Model file for the job. Use its own axes, mm. A direction names the side the tool comes from. Round coordinates to 2 decimals unless told otherwise and drop trailing zeros. Order: outer loops, then holes, each group sorted by start corner. A loop starts at its lowest first (then second) coordinate and runs counter-clockwise, first axis right, second up. Notation, with made-up numbers: (-34.75, 69) - (5.25, 69) arc R4 ccw to (5.25, 75) - close; hole circle Ø2 at (68.5, 19). An arc over 180 degrees is marked (long way). Put each result on its own line as item: value. Start each with the question number.
Item 1: Saw through at B-B on z = -3.5. List the corners of the cut face in (x, y).
Item 2: Mould opens along X. For faces 1 (the face through (-13.268, 9.392, -33.573)), 2 (the face through (32.187, 9.392, -20.386)), 3 (the face through (-36.225, 9.392, -11.806)), 4 (the face through (-11.837, 9.658, -16.703)) say: pulls with the +X half, pulls with the -X half, needs draft (parallel to the pull), parting line crosses it, or undercut.
Item 3: Which spindle directions (+Z, -Z, +X, -X, +Y, -Y) get a long thin tool onto all of the face, cutting with end or side? Do faces 5 (the face through (4.741, 9.392, 37.804)), 6 (the face through (37.1, 9.39, 0.34)), 7 (the face through (32.35, 9.39, 18.17)), 8 (the face through (36.246, 9.392, -11.741)), 9 (the face through (20, 10, -1.9)). Say none if no direction does.
Item 4: Probe probe 1 along Z at (x, y) = (-18, 15.25); probe 2 along Z at (x, y) = (1, 11.5); probe 3 along X at (y, z) = (18, 31.5). List the from-to ranges inside material, lowest first.
Item 5: Pin check, flat tips, straight feed: pin 1 Ø3 at (y, z) = (11.5, -21) entering from -X; pin 2 Ø4 at (x, y) = (21, 13) entering from +Z; pin 3 Ø10 at (y, z) = (15, 20) entering from -X; pin 4 Ø5 at (x, y) = (1, 7.5) entering from +Z. Stop position of each tip, or through.
Item 6: Saw through at A-A on x = 4. List the corners of the cut face in (y, z), plus the area to 3 significant figures.
```python
from build123d import *

# Parameters (mm, degrees)
SKETCH1_R           = 38.1
BOSS_EXTRUDE1_DEPTH = 19.05
CUT_EXTRUDE1_DEPTH  = 33
CIRPATTERN1_COUNT   = 25
SKETCH3_R           = 18
CUT_EXTRUDE2_DEPTH  = 28
CUT_EXTRUDE8_DEPTH  = 23
CIRPATTERN2_COUNT   = 12


with BuildPart() as part:
    # Sketch1 → Boss-Extrude1 (new body)
    with BuildSketch(Plane(origin=(0, 0, 0), x_dir=(1, 0, 0), z_dir=(0, 1, 0))):
        with Locations(Location((0, 0, 0), (0, 0, 90))):
            Circle(SKETCH1_R)
    extrude(amount=BOSS_EXTRUDE1_DEPTH)

    # Sketch2 → Cut-Extrude1 (cut)
    with BuildSketch(Plane.XZ):
        Polygon((0, 38.1), (-2.36, 38.1), (-1.66, 36.1), (0, 36.1), (1.66, 36.1), (2.36, 38.1), align=None)
    cut_extrude1 = extrude(amount=-CUT_EXTRUDE1_DEPTH, mode=Mode.SUBTRACT)

    # CirPattern1: Cut-Extrude1 ×25 about axis
    cirpattern1_axis = Axis((0, 0, 0), (0, 1, 0))
    for i in range(1, CIRPATTERN1_COUNT):
        add(cut_extrude1.rotate(cirpattern1_axis, i * 360 / CIRPATTERN1_COUNT), mode=Mode.SUBTRACT)

    # Sketch3 → Cut-Extrude2 (cut)
    with BuildSketch(Plane(origin=(0, 19.05, 0), x_dir=(1, 0, 0), z_dir=(0, 1, 0))):
        with Locations(Location((0, 0, 0), (0, 0, 270))):
            Circle(SKETCH3_R)
    extrude(amount=-CUT_EXTRUDE2_DEPTH, mode=Mode.SUBTRACT)

    # Sketch3_7 → Cut-Extrude8 (cut)
    with BuildSketch(Plane(origin=(0, 19.05, 0), x_dir=(1, 0, 0), z_dir=(0, 1, 0))):
        with BuildLine():
            Line((0.3, 22.8), (-1.9, 22.8))
            Line((-1.9, 22.8), (-1.9, 17.899441332))
            ThreePointArc((-1.9, 17.899441332), (0.302266808, 17.997461898), (2.5, 17.82554347))
            Line((2.5, 17.82554347), (2.5, 22.8))
            Line((2.5, 22.8), (0.3, 22.8))
        make_face()
    cut_extrude8 = extrude(amount=-CUT_EXTRUDE8_DEPTH, mode=Mode.SUBTRACT)

    # CirPattern2: Cut-Extrude8 ×12 about axis
    cirpattern2_axis = Axis((0, 0, 0), (0, 1, 0))
    for i in range(1, CIRPATTERN2_COUNT):
        add(cut_extrude8.rotate(cirpattern2_axis, i * 360 / CIRPATTERN2_COUNT), mode=Mode.SUBTRACT)


solid = part.part
```
Results found:
1. outline: (-37.94, 0) - (-17.66, 0) - (-17.66, 19.05) - (-37.94, 19.05) - close; (17.66, 0) - (37.94, 0) - (37.94, 19.05) - (17.66, 19.05) - close
2. face 1: undercut
2. face 2: pulls with the +X half
2. face 3: pulls with the -X half
2. face 4: undercut
3. face 5: +Z, +X, +Y, -Y
3. face 6: +X, +Y, -Y
3. face 7: +Z, +Y, -Y
3. face 8: -Z, +X, +Y, -Y
3. face 9: +Y, -Y
4. probe 1: z = -33.58 to -13.28, -8.2 to -2.5, 1.9 to 7.51, 12.59 to 31.3
4. probe 2: z = -38.09 to -22.8, 22.8 to 36.1
4. probe 3: x = -21.43 to -19.59, -17.64 to 17.64, 19.59 to 21.43
5. pin 1: stops at x = -32.73
5. pin 2: stops at z = 32.2
5. pin 3: stops at x = -35.02
5. pin 4: stops at z = 38.03
6. outline: (0, -35.88) - (19.05, -35.88) - (19.05, -17.55) - (0, -17.55) - close; (0, 17.55) - (19.05, 17.55) - (19.05, 37.89) - (0, 37.89) - close
6. area: 737 mm²
